Autodesk Inventor part; units mm, degrees
ref_plane "YZ Plane" through (0, 0, 0) normal (1, 0, 0) x (0, 1, 0)
ref_plane "XZ Plane" through (0, 0, 0) normal (0, 1, 0) x (-1, 0, 0)
ref_plane "XY Plane" through (0, 0, 0) normal (0, 0, 1) x (1, 0, 0)
sketch "RingSketch" plane through (0, 0, 0) normal (0, 0, 1) x (1, 0, 0)
  circle A0 centre (0, 0) radius 10
  dimension "RingDia" = 20
extrude "Ring" add sketch "RingSketch" against normal blind 1
sketch "ShankSketch" plane through (0, 0, -1) normal (0, 0, -1) x (-1, 0, 0)
  circle A0 centre (0, 0) radius 8.975
  dimension "ShankDia" = 17.95
extrude "Shank" add sketch "ShankSketch" along normal blind 10
sketch "ConeSketch" plane through (0, 0, 0) normal (1, 0, 0) x (0, 1, 0)
  line L0 (0, 0) -> (10, 0)
  line L1 (10, 0) -> (5, 8.6603)
  line L2 (5, 8.6603) -> (0, 8.6603)
  line L3 (0, 8.6603) -> (0, 0)
  line L4 (-10, 0) -> (10, 0)
  dimension "ConeAngle" = 60
  dimension "ConeBase" = 10
  dimension "ConeTipDia" = 5
revolve "Cone" add sketch "ConeSketch" angle 360 about axis through (0, 0, 8.6603) along (0, 0, -1)
sketch "SocketSketch" plane through (0, 0, 0) normal (0, 1, 0) x (-1, 0, 0)
  arc A0 (0, 5.6603) -> (0, 15.6603) centre (0, 10.6603) ccw
  line L0 (0, 15.6603) -> (0, 5.6603)
  line L1 (-5, 8.6603) -> (5, 8.6603)
  line L2 (5, 8.6603) -> (10, 0)
  point P0 (0, 0)
  dimension "RecessDia" = 10
  dimension "BallOffset" = 2
revolve "Socket" cut sketch "SocketSketch" angle 360 about axis through (0, 0, 15.6603) along (0, 0, -1)
sketch "MagnetHoleSketch" plane through (0, 0, -11) normal (0, 0, -1) x (-1, 0, 0)
  circle A0 centre (0, 0) radius 4.8
  dimension "MagnetHoleDia" = 9.6
extrude "MagnetHole" cut sketch "MagnetHoleSketch" against normal blind 16.1603
sketch "PartLength" plane through (0, 0, 0) normal (0, 1, 0) x (-1, 0, 0)
  line L0 (-5, 8.6603) -> (5, 8.6603)
  line L1 (-8.975, -11) -> (8.975, -11)
  point P0 (0, 0)
  dimension "PartLen" = 19.6603
equation "\"ConeBase\" = 0.5 * RingDia"
equation "\"ConeTipDia\" = 0.5 * BallDia"
equation "\"RecessDia\" = BallDia"
properties part number "Rod End 20mm Formula-driven"
Could you check a few things on this model? Use its own coordinates, in mm. A direction names the side the tool comes from. Give positions to 0.01 mm unless a question says otherwise; leave off trailing zeros. Loops run counter-clockwise (first coordinate to the right, second up) from the corner with the lowest first, then second, coordinate; pieces in that order, holes last. Notation, with made-up numbers: (-34.5, 58) -> (-3.5, 58) arc R18 ccw to (-3.5, 80) -> close; hole circle Ø8 at (57.5, 65.25). An arc over 180 degrees is marked (long way). Answer as CSV lines item,"result". Start each with the question number.
(1) If we section it at A-A on x = 0: Write out the boundary of the cut face in (y, z) (3 decimals), then the cut area to 3 significant figures.
(2) I need wall thicknesses on probe 1 along Y at (x, z) = (0, 0); probe 2 along Y at (x, z) = (0, -6.5) (3 decimals); probe 3 along X at (y, z) = (2.75, 5). Which ranges of each line are inside material? Lowest first, please.
(3) If we section it at C-C on z = -3.5: Write out the boundary of the cut face in (x, y) (3 decimals), then the cut area to 3 significant figures.
(4) We'd pull the mould along X, two halves only. Please class faces 3 (the flat face through (0, 0, 5.16)), 4 (the conical face through (1.763, 5.597, 7.156)), 5 (the flat face through (-4, -4, -11)): released by +X, released by -X, zero draft, split by the parting line, or undercut.
(5) Which directions (+Z, -Z, +X, -X, +Y, -Y) give clear straight access to the entire face, cutting with the end or side of a thin tool? Please do faces 1 (the cylindrical face through (-2.17, -9.76, -0.49)), 2 (the flat face through (-7, 6, -1)).
(6) I'm going to push flat-ended pins straight in: pin 1 Ø1.5 at (y, z) = (2.5, -4.5) entering from -X; pin 2 Ø10 at (y, z) = (7, -8) entering from +X; pin 3 Ø5 at (x, y) = (1.5, 0) entering from -Z. Where does each tip first touch, or does it pass through?
(7) If we section it at D-D on z = 6: Write out the boundary of the cut face in (x, y), then the cut area to 3 significant figures.
Computed:
1,outline,"(-10, -1) -> (-8.975, -1) -> (-8.975, -11) -> (-4.8, -11) -> (-4.8, 5.16) -> (4.8, 5.16) -> (4.8, -11) -> (8.975, -11) -> (8.975, -1) -> (10, -1) -> (10, 0) -> (5, 8.66) -> (4.583, 8.66) arc R5 cw to (-4.583, 8.66) -> (-5, 8.66) -> (-10, 0) -> close"
1,area,"154 mm2"
2,probe 1,"y = -10 to -4.8, 4.8 to 10"
2,probe 2,"y = -8.975 to -4.8, 4.8 to 8.975"
2,probe 3,"x = -6.56 to -3.93, 3.93 to 6.56"
3,outline,"circle Ø17.95 at (0, 0); hole circle Ø9.6 at (0, 0)"
3,area,"181 mm2"
4,face 3,"undercut"
4,face 4,"split by the parting line"
4,face 5,"zero draft"
5,face 1,"+Z, -Z"
5,face 2,"-Z"
6,pin 1,"stops at x = -8.8"
6,pin 2,"stops at x = 8.75"
6,pin 3,"stops at z = 5.16"
7,outline,"circle Ø13.07 at (0, 0); hole circle Ø3.62 at (0, 0)"
7,area,"124 mm2"
